Autodesk Inventor part; units mm, degrees
ref_plane "YZ Plane" through (0, 0, 0) normal (1, 0, 0) x (0, 1, 0)
ref_plane "XZ Plane" through (0, 0, 0) normal (0, 1, 0) x (-1, 0, 0)
ref_plane "XY Plane" through (0, 0, 0) normal (0, 0, 1) x (1, 0, 0)
sketch "Эскиз6" plane through (0, 0, 0) normal (0, 0, 1) x (1, 0, 0)
  circle A0 centre (0, 0) radius 18
  dimension "d27" = 36
extrude "Выдавливание5" add sketch "Эскиз6" along normal blind 1.9
sketch "Эскиз7" plane through (0, 0, 1.9) normal (0, 0, 1) x (1, 0, 0)
  circle A0 centre (0, 0) radius 16.5
  dimension "d30" = 33
extrude "Выдавливание6" add sketch "Эскиз7" along normal blind 1.35
mirror "Зеркальное отражение1" about plane through (0, 0, 0) normal (0, 0, -1)
sketch "Эскиз8" plane through (0, 0, 3.25) normal (0, 0, 1) x (1, 0, 0)
  circle A0 centre (0, 0) radius 9.75
  dimension "d33" = 19.5
extrude "Выдавливание7" cut sketch "Эскиз8" against normal blind 4
sketch "Эскиз9" plane through (0, 0, -3.25) normal (0, 0, -1) x (-1, 0, 0)
  circle A0 centre (0, 0) radius 9.75
  circle A1 centre (0, 0) radius 6.75 construction
  line L0 (0, -6.75) -> (0, 6.75) construction
  line L1 (-6.75, 0) -> (6.75, 0) construction
  dimension "d44" = 13.5
hole "Отверстие2" at (0, 6.75, -3.25) at (6.75, 0, -3.25) at (-6.75, 0, -3.25) at (0, -6.75, -3.25) direction (0, 0, 1) diameter 3.2 end through all countersink diameter 6 countersink angle 90
properties part number "Колесо D40 под планшайбу"
Here's how the part is built. I have some questions about the finished solid (model axes, mm). A direction names the side the tool comes from. Coordinates: 2 decimals unless noted, no trailing zeros. Order: outer loops, then holes, each group sorted by start corner. A loop starts at its lowest first (then second) coordinate and runs counter-clockwise, first axis right, second up. Notation, with made-up numbers: (55, -34.75) - (83, -34.75) arc R13 ccw to (83, -14.75) - close; hole circle Ø1 at (26.5, -7.75). An arc over 180 degrees is marked (long way). One line per question, with ' | ' between items.
(1) Suppose I cut it at D-D on x = 11. List the corners of the cut face in (y, z) for me, and give its area (3 significant figures).
Report:
outline: (-14.25, -1.9) - (-12.3, -1.9) - (-12.3, -3.25) - (12.3, -3.25) - (12.3, -1.9) - (14.25, -1.9) - (14.25, 1.9) - (12.3, 1.9) - (12.3, 3.25) - (-12.3, 3.25) - (-12.3, 1.9) - (-14.25, 1.9) - close | area: 175 mm2
(2) For faces 5 (the cylindrical face through (15.24, -6.32, -2.57)), 6 (the flat face through (0, 0, -3.25)), 7 (the flat face through (8, -15, 1.9)), which set-ups out of +Z, -Z, +X, -X, +Y, -Y let a thin tool reach every point of the face, with its end or its side?
Report:
face 5: -Z | face 6: -Z, +X, -X, +Y, -Y | face 7: +Z
(3) Suppose I cut it at B-B on x = 6.75. List the corners of the cut face in (y, z) for me.
Report:
outline: (-16.69, -1.9) - (-15.06, -1.9) - (-15.06, -3.25) - (-3, -3.25) - (-1.6, -1.85) - (-1.6, -0.75) - (-7.04, -0.75) - (-7.04, 3.25) - (-15.06, 3.25) - (-15.06, 1.9) - (-16.69, 1.9) - close; (1.6, -1.85) - (3, -3.25) - (15.06, -3.25) - (15.06, -1.9) - (16.69, -1.9) - (16.69, 1.9) - (15.06, 1.9) - (15.06, 3.25) - (7.04, 3.25) - (7.04, -0.75) - (1.6, -0.75) - close
(4) Suppose I cut it at A-A on y = 0. List the corners of the cut face in (x, z) for me, and give its area (3 significant figures).
Report:
outline: (-18, -1.9) - (-16.5, -1.9) - (-16.5, -3.25) - (-9.75, -3.25) - (-8.35, -1.85) - (-8.35, -0.75) - (-9.75, -0.75) - (-9.75, 3.25) - (-16.5, 3.25) - (-16.5, 1.9) - (-18, 1.9) - close; (-5.15, -1.85) - (-3.75, -3.25) - (3.75, -3.25) - (5.15, -1.85) - (5.15, -0.75) - (-5.15, -0.75) - close; (8.35, -1.85) - (9.75, -3.25) - (16.5, -3.25) - (16.5, -1.9) - (18, -1.9) - (18, 1.9) - (16.5, 1.9) - (16.5, 3.25) - (9.75, 3.25) - (9.75, -0.75) - (8.35, -0.75) - close | area: 128 mm2
(5) If we mould it in two halves opening along X, with no side actions, what happens to faces 1 (the cylindrical face through (-2.343, 17.847, 0.027)), 2 (the cylindrical face through (-1.269, 9.667, 1.278)), 3 (the flat face through (7.1, -7.1, 3.25)), 4 (the cylindrical face through (-0.07, 5.15, -1.29))? For each: pulls with the +X half, pulls with the -X half, needs draft (parallel to the pull), parting line crosses it, or undercut.
Report:
face 1: parting line crosses it | face 2: undercut | face 3: needs draft | face 4: undercut
(6) Will these pins go through, and if not, where does the flat tip stop? pin 1 (6 mm diameter, centred on x = 4.5, y = 4.5, fed in from +Z); pin 2 (1.5 mm diameter, centred on y = -13.5, z = 0, fed in from -X); pin 3 (18 mm diameter, centred on x = 2.5, y = -6, fed in from -Z); pin 4 (3.5 mm diameter, centred on x = 0, y = -6.75, fed in from -Z).
Report:
pin 1: stops at z = -0.75 | pin 2: stops at x = -12.71 | pin 3: stops at z = -3.25 | pin 4: stops at z = -2
(7) If I drill on L1, parallel to Y at x = 0, z = -1.25; L2, parallel to Z at x = -5.5, y = -4; L3, parallel to Y at x = 0.5, z = -2.25, over which ranges is the centre line in solid material (lowest first)?
Report:
L1: y = -18 to -8.35, -5.15 to 5.15, 8.35 to 18 | L2: z = -3.25 to -0.75 | L3: y = -16.49 to -8.69, -4.81 to 4.81, 8.69 to 16.49
